The model under review builds one solid part; all positions refer to its coordinate system, in mm. Face numbers are marked on the shaded views. A direction names the side the tool comes from. Coordinates: 2 decimals unless noted, no trailing zeros. Loops run counter-clockwise (first coordinate to the right, second up) from the corner with the lowest first, then second, coordinate; pieces in that order, holes last. Notation, with made-up numbers: (82.25, -16.5) - (86.25, -16.5) arc R32 ccw to (86.25, 21.5) - close; hole circle Ø5 at (-34.5, 66). An arc over 180 degrees is marked (long way). Use a Markdown table: item, result. Add a question column.
1) For the marked faces 4, 5 and 6, list the 3-axis set-ups (+Z, -Z, +X, -X, +Y, -Y) from which the entire face can be reached by the end or side of a thin tool; tool diameter is ignored.
2) The part is to be moulded in two halves that separate along X. For the marked faces 1, 2 and 3, say which applies: pulls with the +X half, pulls with the -X half, needs draft (parallel to the pull), parting line crosses it, or undercut.
3) Add section B-B, the plane z = 0. Give the number of separate pieces and of enclosed holes in the cut face, and give its area (3 significant figures).
4) Clearance check with flat-ended pins moving along their axes: pin 1 (8 mm diameter, centred on x = 71.5, y = -1, fed in from -Z); pin 2 (6.5 mm diameter, centred on x = 98, y = 0, fed in from +Z); pin 3 (1.2 mm diameter, centred on y = -6, z = 0, fed in from +X). State where each tip first meets the part, or that it passes through.
5) Add section C-C, the plane x = 23. Give the boundary of the cut face in (y, z), and give its area (3 significant figures).
6) Add section A-A, the plane x = 98. Give the boundary of the cut face in (y, z), and give its area (3 significant figures).
7) To check wall thickness, follow L1, parallel to X at y = 4.5, z = 0; L2, parallel to Z at x = 90.5, y = 2.75; L3, parallel to X at y = 4.75, z = -5.25. State the ranges of each line that lie inside material, in increasing order. Write a range as [from, to].
Autodesk Inventor part; units mm, degrees
ref_plane "AC_XY" through (98, 0, 0) normal (0, 0, 1) x (1, 0, 0)
ref_plane "AC_YZ" through (98, 0, 0) normal (1, 0, 0) x (0, 1, 0)
ref_plane "AC_ZX" through (98, 0, 0) normal (0, 1, 0) x (0, 0, 1)
sketch "Sketch_2" plane through (0, 0, 0) normal (0, 0, 1) x (1, 0, 0)
  line L0 (106, 0) -> (-12, 0)
  line L1 (87, 0) -> (87, 5)
  line L2 (87, 5) -> (9, 5)
  line L3 (9, 5) -> (9, 2)
  line L4 (9, 2) -> (-12, 2)
  line L5 (-12, 2) -> (-12, 5.233)
  line L6 (-12, 5.233) -> (-11.233, 6)
  line L7 (-11.233, 6) -> (0, 6)
  line L8 (0, 6) -> (0, 7.75)
  line L9 (0, 7.75) -> (0.5, 8.25)
  line L10 (0.5, 8.25) -> (8.5, 8.25)
  line L11 (8.5, 8.25) -> (9, 7.75)
  line L12 (9, 7.75) -> (9, 5.55)
  line L13 (9, 5.55) -> (87, 5.55)
  line L14 (87, 5.55) -> (87, 7.75)
  line L15 (87, 7.75) -> (87.5, 8.25)
  line L16 (87.5, 8.25) -> (91.5, 8.25)
  line L17 (91.5, 8.25) -> (92, 7.75)
  line L18 (92, 7.75) -> (92, 6)
  line L19 (92, 6) -> (105.233, 6)
  line L20 (105.233, 6) -> (106, 5.233)
  line L21 (106, 5.233) -> (106, 0)
  line L22 (106, 0) -> (87, 0)
revolve "Revolution1" add sketch "Sketch_2" angle 360 about axis through (106, 0, 0) along (1, 0, 0)
thread "Thread1"
thread "Thread2"
sketch "Sketch_3" plane through (0, 0, 0) normal (0, 1, 0) x (-1, 0, 0)
  line L0 (-87, 3.45) -> (-87.5, 3.95)
  line L1 (-87.5, 3.95) -> (-96, 3.95)
  line L2 (-96, 3.95) -> (-96, -3.95)
  line L3 (-96, -3.95) -> (-87.5, -3.95)
  line L4 (-87.5, -3.95) -> (-87, -3.45)
  line L5 (-87, -3.45) -> (-87, 3.45)
extrude "Extrusion1" add sketch "Sketch_3" along normal mid plane 16.5
sketch "Sketch_4" plane through (0, 0, 0) normal (0, 1, 0) x (-1, 0, 0)
  line L0 (-92, 13.95) -> (-111, 13.95)
  line L1 (-111, 13.95) -> (-111, -13.95)
  line L2 (-111, -13.95) -> (-92, -13.95)
  line L3 (-92, -13.95) -> (-92, -3.95)
  line L4 (-92, -3.95) -> (-106, -3.95)
  line L5 (-106, -3.95) -> (-106, 3.95)
  line L6 (-106, 3.95) -> (-92, 3.95)
  line L7 (-92, 3.95) -> (-92, 13.95)
extrude "Extrusion2" cut sketch "Sketch_4" along normal mid plane 16.5
sketch "Sketch_5" plane through (0, 0, 0) normal (1, 0, 0) x (0, 1, 0)
  line L0 (-14, 14) -> (-14, -14)
  line L1 (-14, -14) -> (14, -14)
  line L2 (14, -14) -> (14, 14)
  line L3 (14, 14) -> (-14, 14)
  line L4 (-7, 7) -> (-7, -7)
  line L5 (-7, -7) -> (7, -7)
  line L6 (7, -7) -> (7, 7)
  line L7 (7, 7) -> (-7, 7)
extrude "Extrusion3" cut sketch "Sketch_5" along normal blind 9
sketch "Sketch_6" plane through (90.5, 0, 0) normal (1, 0, 0) x (0, 0, -1)
  line L0 (-14, -14) -> (14, -14)
  line L1 (14, -14) -> (14, 14)
  line L2 (14, 14) -> (-14, 14)
  line L3 (-14, 14) -> (-14, -14)
  line L4 (-7, -7) -> (7, -7)
  line L5 (7, -7) -> (7, 7)
  line L6 (7, 7) -> (-7, 7)
  line L7 (-7, 7) -> (-7, -7)
extrude "Extrusion4" cut sketch "Sketch_6" along normal mid plane 18
sketch "Sketch6" plane through (0.5, 7, -4.3661) normal (0, 1, 0) x (1, 0, 0)
  point P0 (5, -4.3661)
hole "Hole1" at (5.5, 7, 0) direction (0, -1, 0) diameter 4.134 depth 7 countersink diameter 5 countersink angle 90
sketch "Sketch7" plane through (91.7124, 7, 3.95) normal (0, 1, 0) x (1, 0, 0)
  point P0 (-1.2124, 3.95)
hole "Hole2" at (90.5, 7, 0) direction (0, -1, 0) diameter 4.134 depth 7 countersink diameter 5 countersink angle 90
sketch "Sketch_9" plane through (0, 0, 0) normal (0, 0, 1) x (1, 0, 0)
  circle A0 centre (98, 0) radius 2
extrude "Extrusion5" cut sketch "Sketch_9" along normal mid plane 7.9
ref_plane "AC_XY" through (98, 0, 0) normal (0, 0, 1) x (1, 0, 0)
ref_plane "AC_YZ" through (98, 0, 0) normal (1, 0, 0) x (0, 1, 0)
ref_plane "AC_ZX" through (98, 0, 0) normal (0, 1, 0) x (0, 0, 1)
ref_plane "DUMMY_XY" through (0, 0, 0) normal (0, 1, 0) x (1, 0, 0)
ref_plane "DUMMY_YZ" through (0, 0, 0) normal (1, 0, 0) x (0, 0, -1)
ref_plane "DUMMY_ZX" through (0, 0, 0) normal (0, 0, -1) x (0, 1, 0)
ref_plane "FM_XY" through (0, 0, 0) normal (-1, 0, 0) x (0, 0, -1)
ref_plane "FM_YZ" through (0, 0, 0) normal (0, 0, -1) x (0, -1, 0)
ref_plane "FM_ZX" through (0, 0, 0) normal (0, -1, 0) x (-1, 0, 0)
ref_plane "FMFM_XY" through (0, 0, 0) normal (-1, 0, 0) x (0, 0, -1)
ref_plane "FMFM_YZ" through (0, 0, 0) normal (0, 0, -1) x (0, -1, 0)
ref_plane "FMFM_ZX" through (0, 0, 0) normal (0, -1, 0) x (-1, 0, 0)
ref_plane "NUT_XY" through (-2, 0, 0) normal (-1, 0, 0) x (0, 0, -1)
ref_plane "NUT_YZ" through (-2, 0, 0) normal (0, 0, -1) x (0, -1, 0)
ref_plane "NUT_ZX" through (-2, 0, 0) normal (0, -1, 0) x (-1, 0, 0)
ref_plane "POINT_XY" through (-12, 0, 0) normal (-1, 0, 0) x (0, 0, -1)
ref_plane "POINT_YZ" through (-12, 0, 0) normal (0, 0, -1) x (0, -1, 0)
ref_plane "POINT_ZX" through (-12, 0, 0) normal (0, -1, 0) x (-1, 0, 0)
ref_plane "RM_XY" through (96, 0, 0) normal (1, 0, 0) x (0, 0, -1)
ref_plane "RM_YZ" through (96, 0, 0) normal (0, 0, -1) x (0, 1, 0)
ref_plane "RM_ZX" through (96, 0, 0) normal (0, 1, 0) x (1, 0, 0)
ref_plane "S_XY" through (26, 0, 0) normal (1, 0, 0) x (0, 0, -1)
ref_plane "S_YZ" through (26, 0, 0) normal (0, 0, -1) x (0, 1, 0)
ref_plane "S_ZX" through (26, 0, 0) normal (0, 1, 0) x (1, 0, 0)
ref_plane "dim_0_XY" through (0, 0, 0) normal (0, 0, 1) x (1, 0, 0)
ref_plane "dim_0_YZ" through (0, 0, 0) normal (1, 0, 0) x (0, 1, 0)
ref_plane "dim_0_ZX" through (0, 0, 0) normal (0, 1, 0) x (0, 0, 1)
ref_plane "dim_bex1_XY" through (105.233, 6, 0) normal (0, 0, 1) x (1, 0, 0)
ref_plane "dim_bex1_YZ" through (105.233, 6, 0) normal (1, 0, 0) x (0, 1, 0)
ref_plane "dim_bex1_ZX" through (105.233, 6, 0) normal (0, 1, 0) x (0, 0, 1)
ref_plane "dim_bex2_XY" through (105.233, -6, 0) normal (0, 0, 1) x (1, 0, 0)
ref_plane "dim_bex2_YZ" through (105.233, -6, 0) normal (1, 0, 0) x (0, 1, 0)
ref_plane "dim_bex2_ZX" through (105.233, -6, 0) normal (0, 1, 0) x (0, 0, 1)
ref_plane "dim_cd1_XY" through (98, 2, 0) normal (0, 0, 1) x (1, 0, 0)
ref_plane "dim_cd1_YZ" through (98, 2, 0) normal (1, 0, 0) x (0, 1, 0)
ref_plane "dim_cd1_ZX" through (98, 2, 0) normal (0, 1, 0) x (0, 0, 1)
ref_plane "dim_cd2_XY" through (98, -2, 0) normal (0, 0, 1) x (1, 0, 0)
ref_plane "dim_cd2_YZ" through (98, -2, 0) normal (1, 0, 0) x (0, 1, 0)
ref_plane "dim_cd2_ZX" through (98, -2, 0) normal (0, 1, 0) x (0, 0, 1)
ref_plane "dim_d1_XY" through (18, 5.55, 0) normal (0, 0, 1) x (1, 0, 0)
ref_plane "dim_d1_YZ" through (18, 5.55, 0) normal (1, 0, 0) x (0, 1, 0)
ref_plane "dim_d1_ZX" through (18, 5.55, 0) normal (0, 1, 0) x (0, 0, 1)
ref_plane "dim_d2_XY" through (18, -5.55, 0) normal (0, 0, 1) x (1, 0, 0)
ref_plane "dim_d2_YZ" through (18, -5.55, 0) normal (1, 0, 0) x (0, 1, 0)
ref_plane "dim_d2_ZX" through (18, -5.55, 0) normal (0, 1, 0) x (0, 0, 1)
ref_plane "dim_ee_XY" through (5.5, 7, 0) normal (0, 0, 1) x (1, 0, 0)
ref_plane "dim_ee_YZ" through (5.5, 7, 0) normal (1, 0, 0) x (0, 1, 0)
ref_plane "dim_ee_ZX" through (5.5, 7, 0) normal (0, 1, 0) x (0, 0, 1)
ref_plane "dim_ee1_XY" through (3, 7, 0) normal (0, 0, 1) x (1, 0, 0)
ref_plane "dim_ee1_YZ" through (3, 7, 0) normal (1, 0, 0) x (0, 1, 0)
ref_plane "dim_ee1_ZX" through (3, 7, 0) normal (0, 1, 0) x (0, 0, 1)
ref_plane "dim_ee2_XY" through (8, 7, 0) normal (0, 0, 1) x (1, 0, 0)
ref_plane "dim_ee2_YZ" through (8, 7, 0) normal (1, 0, 0) x (0, 1, 0)
ref_plane "dim_ee2_ZX" through (8, 7, 0) normal (0, 1, 0) x (0, 0, 1)
ref_plane "dim_ew1_XY" through (96, 0, -3.95) normal (0, 1, 0) x (1, 0, 0)
ref_plane "dim_ew1_YZ" through (96, 0, -3.95) normal (1, 0, 0) x (0, 0, -1)
ref_plane "dim_ew1_ZX" through (96, 0, -3.95) normal (0, 0, -1) x (0, 1, 0)
ref_plane "dim_ew2_XY" through (96, 0, 3.95) normal (0, 1, 0) x (1, 0, 0)
ref_plane "dim_ew2_YZ" through (96, 0, 3.95) normal (1, 0, 0) x (0, 0, -1)
ref_plane "dim_ew2_ZX" through (96, 0, 3.95) normal (0, 0, -1) x (0, 1, 0)
ref_plane "dim_g_XY" through (9, 0, 0) normal (0, 0, 1) x (1, 0, 0)
ref_plane "dim_g_YZ" through (9, 0, 0) normal (1, 0, 0) x (0, 1, 0)
ref_plane "dim_g_ZX" through (9, 0, 0) normal (0, 1, 0) x (0, 0, 1)
ref_plane "dim_gew_bottom_XY" through (-12, -6, 0) normal (0, 0, 1) x (1, 0, 0)
ref_plane "dim_gew_bottom_YZ" through (-12, -6, 0) normal (1, 0, 0) x (0, 1, 0)
ref_plane "dim_gew_bottom_ZX" through (-12, -6, 0) normal (0, 1, 0) x (0, 0, 1)
ref_plane "dim_gew_top_XY" through (-12, 6, 0) normal (0, 0, 1) x (1, 0, 0)
ref_plane "dim_gew_top_YZ" through (-12, 6, 0) normal (1, 0, 0) x (0, 1, 0)
ref_plane "dim_gew_top_ZX" through (-12, 6, 0) normal (0, 1, 0) x (0, 0, 1)
ref_plane "dim_kv41_XY" through (0, 0, 7) normal (1, 0, 0) x (0, 0, -1)
ref_plane "dim_kv41_YZ" through (0, 0, 7) normal (0, 0, -1) x (0, 1, 0)
ref_plane "dim_kv41_ZX" through (0, 0, 7) normal (0, 1, 0) x (1, 0, 0)
ref_plane "dim_kv42_XY" through (0, 0, -7) normal (1, 0, 0) x (0, 0, -1)
ref_plane "dim_kv42_YZ" through (0, 0, -7) normal (0, 0, -1) x (0, 1, 0)
ref_plane "dim_kv42_ZX" through (0, 0, -7) normal (0, 1, 0) x (1, 0, 0)
ref_plane "dim_l_XY" through (92, 6, 0) normal (0, 0, 1) x (1, 0, 0)
ref_plane "dim_l_YZ" through (92, 6, 0) normal (1, 0, 0) x (0, 1, 0)
ref_plane "dim_l_ZX" through (92, 6, 0) normal (0, 1, 0) x (0, 0, 1)
ref_plane "dim_left_XY" through (-12, 0, 0) normal (0, 0, 1) x (1, 0, 0)
ref_plane "dim_left_YZ" through (-12, 0, 0) normal (1, 0, 0) x (0, 1, 0)
ref_plane "dim_left_ZX" through (-12, 0, 0) normal (0, 1, 0) x (0, 0, 1)
ref_plane "dim_right_XY" through (106, 0, 0) normal (0, 0, 1) x (1, 0, 0)
ref_plane "dim_right_YZ" through (106, 0, 0) normal (1, 0, 0) x (0, 1, 0)
ref_plane "dim_right_ZX" through (106, 0, 0) normal (0, 1, 0) x (0, 0, 1)
ref_plane "dim_right_g_XY" through (87, 0, 0) normal (0, 0, 1) x (1, 0, 0)
ref_plane "dim_right_g_YZ" through (87, 0, 0) normal (1, 0, 0) x (0, 1, 0)
ref_plane "dim_right_g_ZX" through (87, 0, 0) normal (0, 1, 0) x (0, 0, 1)
ref_plane "dim_right_hub_XY" through (96, 0, 0) normal (0, 0, 1) x (1, 0, 0)
ref_plane "dim_right_hub_YZ" through (96, 0, 0) normal (1, 0, 0) x (0, 1, 0)
ref_plane "dim_right_hub_ZX" through (96, 0, 0) normal (0, 1, 0) x (0, 0, 1)
ref_plane "dim_va_XY" through (97.5, 0, 0) normal (0, 0, 1) x (1, 0, 0)
ref_plane "dim_va_YZ" through (97.5, 0, 0) normal (1, 0, 0) x (0, 1, 0)
ref_plane "dim_va_ZX" through (97.5, 0, 0) normal (0, 1, 0) x (0, 0, 1)
properties part number "RM/8010/M/50_B0__B"
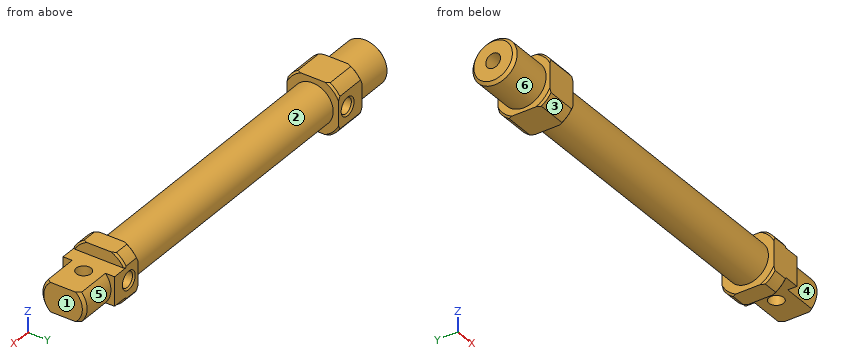
From the geometry:
| question | item | result |
|---|---|---|
| 1 | face 4 | +X, -Y |
| 1 | face 5 | +X, +Y |
| 1 | face 6 | -X |
| 2 | face 1 | pulls with the +X half |
| 2 | face 2 | undercut |
| 2 | face 3 | needs draft |
| 3 | separate pieces | 2 |
| 3 | enclosed holes | 1 |
| 3 | area | 454 mm^2 |
| 4 | pin 1 | stops at z = -5.55 |
| 4 | pin 2 | stops at z = 3.95 |
| 4 | pin 3 | stops at x = 105.83 |
| 5 | outline | circle Ø11.1 at (0, 0); hole circle Ø10 at (0, 0) |
| 5 | area | 18.2 mm^2 |
| 6 | outline | (-4.52, -3.95) - (-2, -3.95) - (-2, 3.95) - (-4.52, 3.95) arc R6 ccw to start; (2, -3.95) - (4.52, -3.95) arc R6 ccw to (4.52, 3.95) - (2, 3.95) - close |
| 6 | area | 55.8 mm^2 |
| 7 | L1 | x = [-12, 3.43], [7.57, 9], [87, 88.43], [92.57, 106] |
| 7 | L2 | z = [-7, -2.07], [2.07, 7] |
| 7 | L3 | x = [0, 9], [87, 92] |
